```python
from build123d import *

# Parameters (mm, degrees)
SKETCH2_R           = 6
BOSS_EXTRUDE1_DEPTH = 8
SKETCH4_R           = 4
BOSS_EXTRUDE2_DEPTH = 25
CUT_EXTRUDE1_DEPTH  = 7


with BuildPart() as part:
    # Sketch2 → Boss-Extrude1 (new body)
    with BuildSketch(Plane(origin=(0, 0, 0), x_dir=(0, 0, -1), z_dir=(1, 0, 0))):
        Circle(SKETCH2_R)
    extrude(amount=BOSS_EXTRUDE1_DEPTH)

    # Sketch4 → Boss-Extrude2 (add)
    with BuildSketch(Plane.ZY):
        Circle(SKETCH4_R)
    extrude(amount=BOSS_EXTRUDE2_DEPTH)

    # Sketch3 → Cut-Extrude1 (cut)
    with BuildSketch(Plane(origin=(8, 0, 0), x_dir=(0, 0, -1), z_dir=(1, 0, 0))):
        Polygon((4, 2.309401077), (0, 4.618802154), (-4, 2.309401077), (-4, -2.309401077), (0, -4.618802154), (4, -2.309401077), align=None)
    extrude(amount=-CUT_EXTRUDE1_DEPTH, mode=Mode.SUBTRACT)


solid = part.part
```
CAD build for the part. Positions are in the model's coordinates, mm. A direction names the side the tool comes from. Round coordinates to 2 decimals unless told otherwise and drop trailing zeros. Order: outer loops, then holes, each group sorted by start corner. A loop starts at its lowest first (then second) coordinate and runs counter-clockwise, first axis right, second up. Notation, with made-up numbers: (-34.5, 10.25) -> (-7.5, 10.25) arc R22 ccw to (-7.5, 48.25) -> close; hole circle Ø10 at (-32, -10). An arc over 180 degrees is marked (long way). Write item = value, one per line.
(1) Pull direction Z, two halves, no side cores. Call faces 1 (the flat face through (0, -3.92, 1.42)), 2 (the flat face through (5, 0, -4)), 3 (the cylindrical face through (-12.325, -3.905, -0.867)), 4 (the flat face through (4.549, -3.448, 2.028)): +Z half, -Z half, draft (parallel to the pull), parting line (faces both ways), or undercut.
Answers follow:
face_1 = draft
face_2 = undercut
face_3 = parting line
face_4 = undercut
(2) Cut at D-D (x = -2.5). Write the cut outline in (y, z).
Answers follow:
outline = circle Ø8 at (0, 0)
(3) Cut at C-C (z = -1.5). Write the cut outline in (x, y).
Answers follow:
outline = (-25, -3.71) -> (0, -3.71) -> (0, -5.81) -> (8, -5.81) -> (8, -3.75) -> (1, -3.75) -> (1, 3.75) -> (8, 3.75) -> (8, 5.81) -> (0, 5.81) -> (0, 3.71) -> (-25, 3.71) -> close
(4) Cut at A-A (x = 2). Write the cut outline in (y, z).
Answers follow:
outline = circle Ø12 at (0, 0); hole (-4.62, 0) -> (-2.31, -4) -> (2.31, -4) -> (4.62, 0) -> (2.31, 4) -> (-2.31, 4) -> close
(5) 3-axis set-ups, long thin cutter, end or side, ignore diameter. For faces 5 (the flat face through (4.549, 3.448, -2.028)), 6 (the cylindrical face through (4, 0, 6)): which of +Z, -Z, +X, -X, +Y, -Y reach the whole face in a straight line?
Answers follow:
face_5 = +X
face_6 = +X, -X
(6) Drill centre lines: L1, parallel to Z at x = 7.5, y = -0.25; L2, parallel to X at y = 1, z = 2.5; L3, parallel to X at y = -4.25, z = -1.5. Where is each one in solid material? Low to high.
Answers follow:
L1 = -5.99 to -4, 4 to 5.99
L2 = -25 to 1
L3 = 0 to 8
(7) Cut at B-B (y = 0). Write the cut outline in (x, z), plus the area to 3 significant figures.
Answers follow:
outline = (-25, -4) -> (0, -4) -> (0, -6) -> (8, -6) -> (8, -4) -> (1, -4) -> (1, 4) -> (8, 4) -> (8, 6) -> (0, 6) -> (0, 4) -> (-25, 4) -> close
area = 240 mm²
(8) Flat gauge pins, fed straight in: P1, Ø2, axis at x = 3, z = -5, coming from the +Y side; P2, Ø6, axis at x = -6.5, y = -0.5, coming from the +Z side. Where does each tip first touch, or does it go through?
Answers follow:
P1 = 4.47
P2 = 4
